Autodesk Inventor part; units mm, degrees
ref_plane "YZ Plane" through (0, 0, 0) normal (1, 0, 0) x (0, 1, 0)
ref_plane "XZ Plane" through (0, 0, 0) normal (0, 1, 0) x (-1, 0, 0)
ref_plane "XY Plane" through (0, 0, 0) normal (0, 0, 1) x (1, 0, 0)
sketch "Sketch1" plane through (0, 0, 0) normal (0, 0, 1) x (1, 0, 0)
  line L0 (3.6662, 6.35) -> (7.3323, 0)
  line L1 (7.3323, 0) -> (3.6662, -6.35)
  line L2 (3.6662, -6.35) -> (-3.6662, -6.35)
  line L3 (-3.6662, -6.35) -> (-7.3323, 0)
  line L4 (-7.3323, 0) -> (-3.6662, 6.35)
  line L5 (-3.6662, 6.35) -> (3.6662, 6.35)
  circle A0 centre (0, 0) radius 25.4
  circle A1 centre (0, 0) radius 7.3323 construction
  dimension "d0" = 12.7
  dimension "d2" = 50.8
  dimension "d3" = 18.0677
extrude "Extrusion1" add sketch "Sketch1" against normal blind 4.7625
properties part number "1_2x2x1_4-hexBearing" material "PC/ABS Plastic"
Could you check a few things on this model? Use its own coordinates, in mm. A direction names the side the tool comes from. Coordinates: 2 decimals unless noted, no trailing zeros. Order: outer loops, then holes, each group sorted by start corner. A loop starts at its lowest first (then second) coordinate and runs counter-clockwise, first axis right, second up. Notation, with made-up numbers: M 34.5,86 L 77.5,86 A10 cw 77.5,102 Z; hole C 24.5,46.5 d8. An arc over 180 degrees is marked long. Use a Markdown table: item, result. Add a question column.
Q1. Which directions (+Z, -Z, +X, -X, +Y, -Y) give clear straight access to the entire face, cutting with the end or side of a thin tool? Please do faces 4 (the flat face through (5.525, -3.131, -2.348)), 5 (the flat face through (5, -5, -4.762)).
Q2. I'm going to push flat-ended pins straight in: pin 1 (2 mm diameter, centred on y = 6, z = -1, fed in from +X); pin 2 (2 mm diameter, centred on x = 17, z = -3, fed in from -Y); pin 3 (2 mm diameter, centred on x = -0.5, z = -3.5, fed in from -Y). Where does each tip first touch, or does it pass through?
Q3. We'd pull the mould along X, two halves only. Please class faces 1 (the cylindrical face through (-5.506, -24.796, -2.348)), 2 (the flat face through (0, -6.35, -2)), 3 (the flat face through (5, -5, 0)): pulls with the +X half, pulls with the -X half, needs draft (parallel to the pull), parting line crosses it, or undercut.
Q4. I want a section at D-D on x = 21.5. List the corners of the cut face in (y, z) for me.
Q5. I want a section at B-B on y = -1.5. List the corners of the cut face in (x, z) for me.
Q6. I want a section at A-A on x = 0. List the corners of the cut face in (y, z) for me, then the cut area to 3 significant figures.
Q7. I want a section at C-C on z = -3.5. List the corners of the cut face in (x, y) for me, then the cut area to 3 significant figures.
Q8. If I drill on L1, parallel to Y at x = 0.5, z = -1.3; L2, parallel to Y at x = -6, z = -1.65; L3, parallel to X at y = 5.5, z = -1.1, over which ranges is the centre line in solid material (lowest first)?
Checked values:
| question | item | result |
|---|---|---|
| 1 | face 4 | +Z, -Z |
| 1 | face 5 | -Z, +X, -X, +Y, -Y |
| 2 | pin 1 | x = 24.9 |
| 2 | pin 2 | y = -19.73 |
| 2 | pin 3 | y = -25.4 |
| 3 | face 1 | parting line crosses it |
| 3 | face 2 | undercut |
| 3 | face 3 | needs draft |
| 4 | outline | M -13.52,-4.76 L 13.52,-4.76 L 13.52,0 L -13.52,0 Z |
| 5 | outline | M -25.36,-4.76 L -6.47,-4.76 L -6.47,0 L -25.36,0 Z; M 6.47,-4.76 L 25.36,-4.76 L 25.36,0 L 6.47,0 Z |
| 6 | outline | M -25.4,-4.76 L -6.35,-4.76 L -6.35,0 L -25.4,0 Z; M 6.35,-4.76 L 25.4,-4.76 L 25.4,0 L 6.35,0 Z |
| 6 | area | 181 mm² |
| 7 | outline | C 0,0 d50.8; hole M -7.33,0 L -3.67,-6.35 L 3.67,-6.35 L 7.33,0 L 3.67,6.35 L -3.67,6.35 Z |
| 7 | area | 1,890 mm² |
| 8 | L1 | -25.4 to -6.35, 6.35 to 25.4 |
| 8 | L2 | -24.68 to -2.31, 2.31 to 24.68 |
| 8 | L3 | -24.8 to -4.16, 4.16 to 24.8 |
